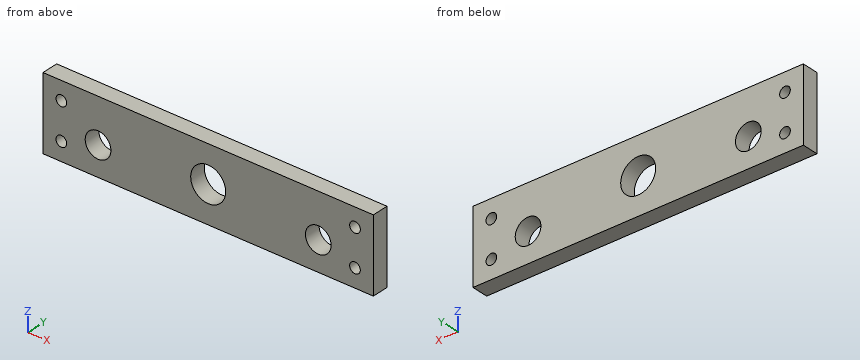
from build123d import *

# Parameters (mm, degrees)
SKETCH1_R           = 1.45
BOSS_EXTRUDE1_DEPTH = 4.5
SKETCH2_R           = 3.5
CUT_EXTRUDE1_DEPTH  = 5.5


with BuildPart() as part:
    # Sketch1 → Boss-Extrude1 (new body)
    with BuildSketch(Plane(origin=(0, 0, 0), x_dir=(1, 0, 0), z_dir=(0, 1, 0))):
        with BuildLine():
            Line((0, 4.7625), (0, 10))
            Line((0, 10), (-45, 10))
            Line((-45, 10), (-45, -10))
            Line((-45, -10), (0, -10))
            Line((0, -10), (0, -4.7625))
            ThreePointArc((0, -4.7625), (-4.7625, 0), (0, 4.7625))
        make_face()
        with Locations((-40, 5)):
            Circle(SKETCH1_R, mode=Mode.SUBTRACT)
        with Locations((-40, -5)):
            Circle(SKETCH1_R, mode=Mode.SUBTRACT)
    boss_extrude1 = extrude(amount=BOSS_EXTRUDE1_DEPTH)

    # Mirror1: Boss-Extrude1 across plane
    add(boss_extrude1.mirror(Plane(origin=(0, 4.5, 10), x_dir=(0, 0, 1), z_dir=(-1, 0, 0))))

    # Sketch2 → Cut-Extrude1 (cut, through all)
    with BuildSketch(Plane(origin=(0, 4.5, 0), x_dir=(1, 0, 0), z_dir=(0, 1, 0))):
        with Locations((-30, 2)):
            Circle(SKETCH2_R)
        with Locations((30, 2)):
            Circle(SKETCH2_R)
    extrude(amount=-CUT_EXTRUDE1_DEPTH, mode=Mode.SUBTRACT)


solid = part.part
Build history of the part. All positions in model axes, mm. Give positions to 0.01 mm unless a question says otherwise; leave off trailing zeros. Write each loop counter-clockwise with the first axis right and the second up, starting at its lowest first coordinate (ties: lowest second). Pieces come first, ordered by that corner, then holes. Notation, with made-up numbers: (81.25, 87.5) - (109.25, 87.5) arc R35 cw to (109.25, 124.5) - close; hole circle Ø10 at (43, 74.25). An arc over 180 degrees is marked (long way). Use one line per item in the form item = value. Start each with the question number.
1. Band-saw the part on A-A on x = 30. Write the cut outline in (y, z), plus the area to 3 significant figures.
2. Band-saw the part on C-C on z = -2. Write the cut outline in (x, y), plus the area to 3 significant figures.
3. Band-saw the part on B-B on x = -40. Write the cut outline in (y, z), plus the area to 3 significant figures.
4. Probe line 1 (Z direction, x = 40, y = 2.5); line 2 (Z direction, x = -30, y = 1); line 3 (X direction, y = 2.5, z = -5). List the from-to ranges inside material, lowest first. Write a range as [from, to].
5. Drop a flat-ended pin along its axis: pin 1 Ø6.5 at (x, z) = (-30, -2) entering from +Y. Give the stop position or say it passes through.
6. Band-saw the part on D-D on y = 1.25. Count the separate pieces of the cut face and the enclosed holes in it, plus the area to 3 significant figures.
Conclusion:
q1.outline = (0, -10) - (4.5, -10) - (4.5, -5.5) - (0, -5.5) - close; (0, 1.5) - (4.5, 1.5) - (4.5, 10) - (0, 10) - close
q1.area = 58.5 mm²
q2.outline = (-45, 0) - (-33.5, 0) - (-33.5, 4.5) - (-45, 4.5) - close; (-26.5, 0) - (-4.32, 0) - (-4.32, 4.5) - (-26.5, 4.5) - close; (4.32, 0) - (26.5, 0) - (26.5, 4.5) - (4.32, 4.5) - close; (33.5, 0) - (45, 0) - (45, 4.5) - (33.5, 4.5) - close
q2.area = 303 mm²
q3.outline = (0, -10) - (4.5, -10) - (4.5, -6.45) - (0, -6.45) - close; (0, -3.55) - (4.5, -3.55) - (4.5, 3.55) - (0, 3.55) - close; (0, 6.45) - (4.5, 6.45) - (4.5, 10) - (0, 10) - close
q3.area = 63.9 mm²
q4.line_1 = [-10, -6.45], [-3.55, 3.55], [6.45, 10]
q4.line_2 = [-10, -5.5], [1.5, 10]
q4.line_3 = [-45, -41.45], [-38.55, -31.8], [-28.2, 28.2], [31.8, 38.55], [41.45, 45]
q5.pin_1 = through
q6.separate_pieces = 1
q6.enclosed_holes = 7
q6.area = 1,630 mm²
